from build123d import *

# Parameters (mm, degrees)
F0_R     = 1.6002
F1_DEPTH = 3.2004


# Not quite as in the source:
# - ends of sketch curves that miss each other by under 0.0002 mm in the source are joined


with BuildPart() as f1:
    # F0 (on Top) → F1 (new body)
    with BuildSketch(Plane.XY):
        with BuildLine():
            ThreePointArc((-4.1050543049, 1.270002348), (-5.3326449309, 1.5185429247), (-6.3685964739, 2.2225))
            ThreePointArc((-6.3685964739, 2.2225), (-11.811, 0), (-6.3685964739, -2.2225))
            ThreePointArc((-6.3685964739, -2.2225), (-5.3326449309, -1.5185429247), (-4.1050543049, -1.270002348))
            Line((-4.1050543049, -1.270002348), (-4.1011929479, -1.27))
            Line((-4.1011929479, -1.27), (5.0438975516, -1.27))
            ThreePointArc((5.0438975516, -1.27), (6.1022308849, -1.451581293), (7.0395100229, -1.9755555556))
            ThreePointArc((7.0395100229, -1.9755555556), (11.176, 0), (7.0395100229, 1.9755555556))
            ThreePointArc((7.0395100229, 1.9755555556), (6.1022308849, 1.451581293), (5.0438975516, 1.27))
            Line((5.0438975516, 1.27), (-4.1011929479, 1.27))
            Line((-4.1011929479, 1.27), (-4.1050543049, 1.270002348))
        make_face()
        with Locations((-8.636, 0)):
            Circle(F0_R, mode=Mode.SUBTRACT)
        with Locations((8.636, 0)):
            Circle(F0_R, mode=Mode.SUBTRACT)
    extrude(amount=F1_DEPTH)


solid = f1.part
Work out the finished part from the listing and answer in its coordinate system (mm). A direction names the side the tool comes from. Coordinates: 2 decimals unless noted, no trailing zeros. Write each loop counter-clockwise with the first axis right and the second up, starting at its lowest first coordinate (ties: lowest second). Pieces come first, ordered by that corner, then holes.
1. Consider line 1 along X through (y, z) = (0.75, 1.2); line 2 along X through (y, z) = (-0.5, 1.55); line 3 along Y through (x, z) = (3, 1.1). Determine where each line is inside the solid, lowest interval first.
Results list:
line 1: x = -11.72 to -10.05, -7.22 to 7.22, 10.05 to 11.06
line 2: x = -11.77 to -10.16, -7.12 to 7.12, 10.16 to 11.13
line 3: y = -1.27 to 1.27
2. The part is cut by section A-A, the plane y = 0. Write down the section's boundary in (x, z), and give its area (3 significant figures).
Results list:
outline: (-11.81, 0) - (-10.24, 0) - (-10.24, 3.2) - (-11.81, 3.2) - close; (-7.04, 0) - (7.04, 0) - (7.04, 3.2) - (-7.04, 3.2) - close; (10.24, 0) - (11.18, 0) - (11.18, 3.2) - (10.24, 3.2) - close
area: 53.1 mm2
3. The part is cut by section C-C, the plane z = 0.3. State how many separate pieces and enclosed holes the cut face has, and give its area (3 significant figures).
Results list:
separate pieces: 1
enclosed holes: 2
area: 66.8 mm2
4. Flat-ended cylindrical pins translate along their axes: pin 1 (1 mm diameter, centred on x = -6, y = -2, fed in from -Z); pin 2 (1 mm diameter, centred on x = 1, z = 2, fed in from +Y); pin 3 (1 mm diameter, centred on x = 0.5, z = 1, fed in from -Y). Find the tip coordinate at first contact, or state that the pin passes through.
Results list:
pin 1: stops at z = 0
pin 2: stops at y = 1.27
pin 3: stops at y = -1.27
5. For a pull along Y with two mould halves and no side action, classify faces 1 (the flat face through (0, 0, 0)), 2 (the cylindrical face through (11.175, -0.08, 1.578)), 3 (the cylindrical face through (10.162, 0.481, 1.578)) as +Y half, -Y half, draft (parallel to the pull), parting line (faces both ways), or undercut.
Results list:
face 1: draft
face 2: parting line
face 3: undercut
6. The part is cut by section D-D, the plane x = -2.75. Write down the section's boundary in (y, z), and give its area (3 significant figures).
Results list:
outline: (-1.27, 0) - (1.27, 0) - (1.27, 3.2) - (-1.27, 3.2) - close
area: 8.13 mm2
7. For faces 4 (the cylindrical face through (6.088, -1.447, 1.578)), 5 (the cylindrical face through (6.12, 1.46, 1.58)), 6 (the cylindrical face through (-10.235, 0.07, 1.578)), determine the directions among +Z, -Z, +X, -X, +Y, -Y from which every point of the face is accessible in a straight line to the end or side of a thin tool.
Results list:
face 4: +Z, -Z, -Y
face 5: +Z, -Z, +Y
face 6: +Z, -Z
8. The part is cut by section B-B, the plane x = 9.5. Write down the section's boundary in (y, z).
Results list:
outline: (-2.39, 0) - (-1.35, 0) - (-1.35, 3.2) - (-2.39, 3.2) - close; (1.35, 0) - (2.39, 0) - (2.39, 3.2) - (1.35, 3.2) - close
